from build123d import *

# Parameters (mm, degrees)
F1_DEPTH = 63.5
F2_DEPTH = 25.4
F3_DEPTH = 7.9375
F5_R     = 6.35


with BuildPart() as f1:
    # F0 (on Front) → F1 (new body, symmetric)
    with BuildSketch(Plane.XZ):
        Polygon((-41.275, 9.525), (-41.275, -9.525), (41.275, -9.525), (41.275, 9.525), (22.225, 9.525), align=None)
    extrude(amount=F1_DEPTH, both=True)

    # F0 (on Front) → F2 (join, symmetric)
    with BuildSketch(Plane.XZ):
        with BuildLine():
            Line((22.225, 9.525), (41.275, 9.525))
            Line((41.275, 9.525), (41.275, 31.257566))
            ThreePointArc((41.275, 31.257566), (42.593834, 37.59268), (46.33121, 42.8752))
            Line((46.33121, 42.8752), (60.325, 42.8752))
            Line((60.325, 42.8752), (60.325, 61.9252))
            Line((60.325, 61.9252), (40.43917, 61.9252))
            ThreePointArc((40.43917, 61.9252), (27.121835, 49.091941), (22.225, 31.257566))
            Line((22.225, 31.257566), (22.225, 9.525))
        make_face()
    extrude(amount=F2_DEPTH, both=True)

    # F0 (on Front) → F3 (join, symmetric)
    with BuildSketch(Plane.XZ):
        with BuildLine():
            add(Edge.make_bspline(
                [(-41.275, 9.525), (-41.567614, 43.979483), (5.612445, 61.028755), (40.43917, 61.9252)],
                knots=[0, 0, 0, 0, 97.072068, 97.072068, 97.072068, 97.072068], degree=3))
            Line((-41.275, 9.525), (22.225, 9.525))
            Line((22.225, 9.525), (22.225, 31.257566))
            ThreePointArc((22.225, 31.257566), (27.121835, 49.091941), (40.43917, 61.9252))
        make_face()
    extrude(amount=F3_DEPTH, both=True)

    # F0 (on Front) → F4 (revolve)
    with BuildSketch(Plane.XZ):
        Polygon((60.325, 66.675), (60.325, 61.9252), (77.771246, 61.9252), (77.771246, 42.8752), (60.325, 42.8752), (60.325, 38.1), (111.125, 38.1), (111.125, 66.675), align=None)
    revolve(axis=Axis((60.325, 0, 52.3875), (0, 0, 1)))

    # F5
    f5_edges = [f1.edges().sort_by_distance(p)[0] for p in [
        (-41.275, -63.5, 0),
        (41.275, -63.5, 0),
        (41.275, 63.5, 0),
        (-41.275, 63.5, 0),
    ]]
    fillet(f5_edges, radius=F5_R)


solid = f1.part
Geometry check sheet. Reference: the model listing, model coordinates, mm. A direction names the side the tool comes from. Round coordinates to 2 decimals unless told otherwise and drop trailing zeros. Write each loop counter-clockwise with the first axis right and the second up, starting at its lowest first coordinate (ties: lowest second). Pieces come first, ordered by that corner, then holes. Notation, with made-up numbers: (-7.5, -7) -> (43.5, -7) arc R16 ccw to (43.5, 8) -> close; hole circle Ø8 at (65, 37). An arc over 180 degrees is marked (long way). One line per item, written item: value. Start each with the question number.
(1) Scan lines: line 1 (Z direction, x = 20.5, y = -50.5) (3 decimals); line 2 (Y direction, x = -26.5, z = 16.5); line 3 (Y direction, x = 40.5, z = 33). Record each from-to range of solid material in increasing order. Write a range as [from, to].
(2) Cross-section at A-A, the plane z = 3. Record the cut outline in (x, y) (3 decimals).
(3) Go/stop test with flat-tipped pins: pin 1 Ø2 at (x, y) = (79, -15) entering from -Z; pin 2 Ø1 at (x, z) = (93, 42) entering from -Y; pin 3 Ø10.5 at (x, z) = (29, 18) entering from -Y; pin 4 Ø21 at (y, z) = (0.5, 55) entering from +X (3 decimals). Record where each tip stops, or that it passes through.
(4) Draft check along X on faces 4 (the cylindrical face through (107.25, -19.46, 52.59)), 5 (the cylindrical face through (-39.464, 61.59, -0.133)), 6 (the flat face through (60.325, 0, 52)). Enter one of: +X half, -X half, draft (parallel to the pull), parting line (faces both ways), or undercut.
(5) Access from +Z, -Z, +X, -X, +Y, -Y to the whole of each face (thin tool, end or side, straight path). Record for faces 1 (the flat face through (1, 35, 9.525)), 2 (the flat face through (32, 25.4, 24)), 3 (the flat face through (41.275, -1, 6)).
(6) Cross-section at D-D, the plane x = 88.5. Record the cut outline in (y, z) (3 decimals).
(7) Cross-section at B-B, the plane x = 63. Record the cut outline in (y, z) (3 decimals).
(8) Cross-section at C-C, the plane y = 32. Record the cut outline in (x, z) (3 decimals), and give its area (3 significant figures).
Answer:
1. line 1: [-9.525, 9.525]
1. line 2: [-7.94, 7.94]
1. line 3: [-25.4, 25.4]
2. outline: (-41.275, -57.15) arc R6.35 ccw to (-34.925, -63.5) -> (34.925, -63.5) arc R6.35 ccw to (41.275, -57.15) -> (41.275, 57.15) arc R6.35 ccw to (34.925, 63.5) -> (-34.925, 63.5) arc R6.35 ccw to (-41.275, 57.15) -> close
3. pin 1: z = 38.1
3. pin 2: y = -39.31
3. pin 3: y = -25.4
3. pin 4: x = 111.125
4. face 4: parting line
4. face 5: -X half
4. face 6: undercut
5. face 1: -X, +Y
5. face 2: +X, -X, +Y
5. face 3: -Z, +X, +Y, -Y
6. outline: (-42.271, 38.1) -> (42.271, 38.1) -> (42.271, 66.675) -> (-42.271, 66.675) -> close
7. outline: (-50.73, 38.1) -> (50.73, 38.1) -> (50.73, 66.675) -> (-50.73, 66.675) -> close; hole (-17.24, 42.875) -> (17.24, 42.875) -> (17.24, 61.925) -> (-17.24, 61.925) -> close
8. outline: (-41.275, -9.525) -> (41.275, -9.525) -> (41.275, 9.525) -> (-41.275, 9.525) -> close; (20.871, 38.1) -> (99.779, 38.1) -> (99.779, 66.675) -> (20.871, 66.675) -> close
8. area: 3,830 mm²
